Job drawing, mm, ordinate dimensions from the low corner. One solid piece. Round coordinates to 2 decimals unless told otherwise and drop trailing zeros. Write each loop counter-clockwise with the first axis right and the second up, starting at its lowest first coordinate (ties: lowest second). Pieces come first, ordered by that corner, then holes.
1) Saw through at A-A (y = 34.5). Write the cut outline in (x, z) (3 decimals), plus the area to 3 significant figures.
2) Wall check: probe 1 along Y at (x, z) = (30.5, 0.45); probe 2 along X at (y, z) = (22, 1.25) (3 decimals); probe 3 along Y at (x, z) = (10.5, 0.45). Give the ranges that are in metal, low to high.
3) Saw through at B-B (x = 35). Write the cut outline in (y, z), plus the area to 3 significant figures.
4) Flat gauge pins, fed straight in: pin 1 (0.6 mm diameter, centred on x = 1, z = 1, fed in from -Y); pin 2 (1 mm diameter, centred on x = 52.5, z = 1, fed in from -Y); pin 3 (0.6 mm diameter, centred on y = 20, z = 0.5, fed in from +X). Where does each tip first touch, or does it go through?
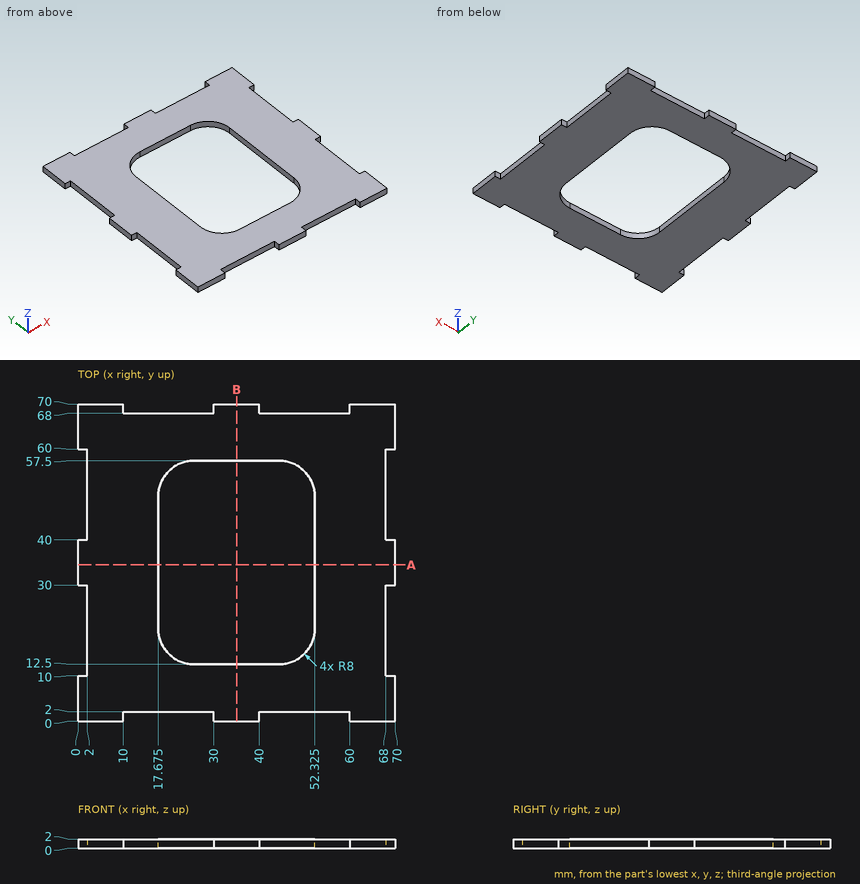
Evaluation:
1. outline: (0, 0) - (17.675, 0) - (17.675, 2) - (0, 2) - close; (52.325, 0) - (70, 0) - (70, 2) - (52.325, 2) - close
1. area: 70.7 mm2
2. probe 1: y = 0 to 12.5, 57.5 to 70
2. probe 2: x = 2 to 17.675, 52.325 to 68
2. probe 3: y = 2 to 68
3. outline: (0, 0) - (12.5, 0) - (12.5, 2) - (0, 2) - close; (57.5, 0) - (70, 0) - (70, 2) - (57.5, 2) - close
3. area: 50.0 mm2
4. pin 1: stops at y = 0
4. pin 2: stops at y = 2
4. pin 3: stops at x = 68
